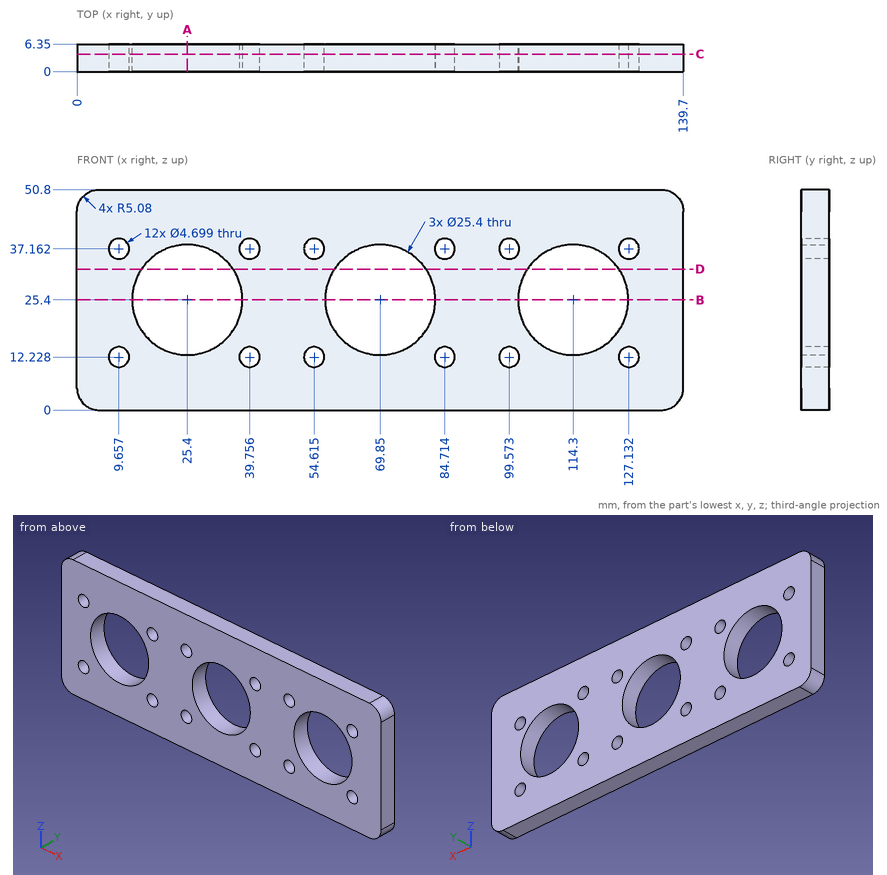
Study the drawing (mm; zero at the part's minimum x, y, z) and answer. Coordinates: 2 decimals unless noted, no trailing zeros. Order: outer loops, then holes, each group sorted by start corner. A loop starts at its lowest first (then second) coordinate and runs counter-clockwise, first axis right, second up. Notation, with made-up numbers: (46.25, 57.25) -> (86.25, 57.25) arc R11 ccw to (86.25, 72.25) -> close; hole circle Ø2 at (79.25, 52.5). An arc over 180 degrees is marked (long way). Answer in a Markdown table with one row per item. Add a question column.
Item 1: Find section A-A (x = 25.4). Write down the section's boundary in (y, z), then the cut area to 3 significant figures.
Item 2: Find the intervals of material crossed by L1, parallel to Z at x = 99.5, y = 2.75; L2, parallel to Z at x = 114.5, y = 5.75; L3, parallel to X at y = 4.25, z = 18, in increasing order. Write a range as from..to.
Item 3: This flat-tipped pin is pushed along its axis until it touches: P1, Ø4, axis at x = 99.57, z = 12.23, coming from the -Y side. Where does it stop, or does it pass through?
Item 4: Find section B-B (z = 25.4). Write down the section's boundary in (x, y).
Item 5: Find section D-D (z = 32.5). Write down the section's boundary in (x, y).
Item 6: Find section C-C (y = 4). State how many separate pieces and enclosed holes the cut face has, then the cut area to 3 significant figures.
Result set:
| question | item | result |
|---|---|---|
| 1 | outline | (0, 0) -> (6.35, 0) -> (6.35, 12.7) -> (0, 12.7) -> close; (0, 38.1) -> (6.35, 38.1) -> (6.35, 50.8) -> (0, 50.8) -> close |
| 1 | area | 161 mm² |
| 2 | L1 | z = 0..9.88, 14.58..34.81, 39.51..50.8 |
| 2 | L2 | z = 0..12.7, 38.1..50.8 |
| 2 | L3 | x = 0..15.08, 35.72..59.53, 80.17..103.98, 124.62..139.7 |
| 3 | P1 | passes through |
| 4 | outline | (0, 0) -> (12.7, 0) -> (12.7, 6.35) -> (0, 6.35) -> close; (38.1, 0) -> (57.15, 0) -> (57.15, 6.35) -> (38.1, 6.35) -> close; (82.55, 0) -> (101.6, 0) -> (101.6, 6.35) -> (82.55, 6.35) -> close; (127, 0) -> (139.7, 0) -> (139.7, 6.35) -> (127, 6.35) -> close |
| 5 | outline | (0, 0) -> (14.87, 0) -> (14.87, 6.35) -> (0, 6.35) -> close; (35.93, 0) -> (59.32, 0) -> (59.32, 6.35) -> (35.93, 6.35) -> close; (80.38, 0) -> (103.77, 0) -> (103.77, 6.35) -> (80.38, 6.35) -> close; (124.83, 0) -> (139.7, 0) -> (139.7, 6.35) -> (124.83, 6.35) -> close |
| 6 | separate pieces | 1 |
| 6 | enclosed holes | 15 |
| 6 | area | 5,350 mm² |
